from build123d import *

# Parameters (mm, degrees)
F0_W      = 43
F0_H      = 79
F0_W_2    = 28
F0_H_2    = 64
F1_DEPTH  = 22
F2_W      = 26
F2_H      = 10.2
F2_H_2    = 1.8
F2_H_3    = 5
F2_W_2    = 1
F3_DEPTH  = 100
F4_R      = 1.75
F5_DEPTH  = 100
F4_R_2    = 3
F6_DEPTH  = 2
F7_R      = 1.75
F8_DEPTH  = 2
F9_W      = 8.5
F9_H      = 20
F10_DEPTH = 20
F11_R     = 3
F12_DEPTH = 25
F13_SIZE  = 2
F14_R     = 5
F15_R     = 2


# Not quite as in the source:
# - a feature names something its author has since deleted; it is built from what else it names


with BuildPart() as f1:
    # F0 (on Top) → F1 (new body)
    with BuildSketch(Plane.XY):
        Rectangle(F0_W, F0_H)
        Rectangle(F0_W_2, F0_H_2, mode=Mode.SUBTRACT)
        Rectangle(F0_W_2, F0_H_2)
    extrude(amount=F1_DEPTH)

    # F2 (on face) → F3 (cut)
    with BuildSketch(Plane.XZ.offset(39.5)):
        with Locations((0, 16.9)):
            Rectangle(F2_W, F2_H)
        with Locations((0, 10.9)):
            Rectangle(F2_W, F2_H_2)
        with Locations((0, 7.5)):
            Rectangle(F2_W, F2_H_3)
        with Locations((-13.5, 10.9)):
            Rectangle(F2_W_2, F2_H_2)
        with Locations((13.5, 10.9)):
            Rectangle(F2_W_2, F2_H_2)
    extrude(amount=-F3_DEPTH, mode=Mode.SUBTRACT)

    # F4 (on face) → F5 (cut)
    with BuildSketch(Plane(origin=(-21.5, 0, 0), x_dir=(0, -1, 0), z_dir=(-1, 0, 0))):
        with Locations((16.5, 17)):
            Circle(F4_R)
    extrude(amount=-F5_DEPTH, mode=Mode.SUBTRACT)

    # F4 (on face) → F6 (cut)
    with BuildSketch(Plane(origin=(-21.5, 0, 0), x_dir=(0, -1, 0), z_dir=(-1, 0, 0))):
        with Locations((16.5, 17)):
            Circle(F4_R_2)
        with Locations((16.5, 17)):
            Circle(F4_R, mode=Mode.SUBTRACT)
    extrude(amount=-F6_DEPTH, mode=Mode.SUBTRACT)

    # F7 (on face) → F8 (cut)
    with BuildSketch(Plane.YZ.offset(21.5)):
        Polygon((-18.2320508076, 14), (-14.7679491924, 14), (-13.0358983849, 17), (-14.7679491924, 20), (-18.2320508076, 20), (-19.9641016151, 17), align=None)
        with Locations((-16.5, 17)):
            Circle(F7_R, mode=Mode.SUBTRACT)
    extrude(amount=-F8_DEPTH, mode=Mode.SUBTRACT)

    # F9 (on face) → F10 (join)
    with BuildSketch(Plane.XY.offset(22)):
        with Locations((17.25, -2.5)):
            Rectangle(F9_W, F9_H)
    extrude(amount=F10_DEPTH)

    # F11 (on face) → F12 (cut)
    with BuildSketch(Plane.YZ.offset(21.5)):
        with Locations((-2.5, 32)):
            Circle(F11_R)
    extrude(amount=-F12_DEPTH, mode=Mode.SUBTRACT)

    # F13
    f13_edges = [f1.edges().sort_by_distance(p)[0] for p in [
        (13, -5.5, 32),
    ]]
    chamfer(f13_edges, length=F13_SIZE)

    # F14
    f14_edges = [f1.edges().sort_by_distance(p)[0] for p in [
        (17.25, 7.5, 42),
        (17.25, -12.5, 42),
        (17.25, -12.5, 22),
        (17.25, 7.5, 22),
        (17.25, 39.5, 22),
        (17.25, -39.5, 22),
        (-17.25, -39.5, 22),
        (-17.25, 39.5, 22),
    ]]
    fillet(f14_edges, radius=F14_R)

    # F15
    f15_edges = [f1.edges().sort_by_distance(p)[0] for p in [
        (13, 0, 5),
        (-13, 0, 5),
        (21.5, 0, 0),
        (-21.5, 0, 0),
    ]]
    fillet(f15_edges, radius=F15_R)


solid = f1.part
Design review of the part built by this model. Coordinates are the model's own, in mm. A direction names the side the tool comes from. Round coordinates to 2 decimals unless told otherwise and drop trailing zeros. Write each loop counter-clockwise with the first axis right and the second up, starting at its lowest first coordinate (ties: lowest second). Pieces come first, ordered by that corner, then holes.
Item 1: Consider section B-B on z = 32. Give the boundary of the cut face in (x, y).
Item 2: Draft analysis for pull direction Z (two halves, no side actions). For faces 1 (the cylindrical face through (17.31, 6, 40.57)), 2 (the cylindrical face through (16.205, -16.272, 18.735)), 3 (the flat face through (-13, -1, 9)), state which applies: released by +Z, released by -Z, zero draft, split by the parting line, or undercut.
Item 3: Consider section C-C on x = -18. Give the boundary of the cut face in (y, z), and give its area (3 significant figures).
Item 4: For faces 4 (the flat face through (17, -26, 22)), 5 (the cylindrical face through (-20.5, -14.1, 15.2)), 6 (the cylindrical face through (-12.4, 0.55, 5.57)), 7 (the flat face through (19.5, -15, 15.7)), list the 3-axis set-ups (+Z, -Z, +X, -X, +Y, -Y) from which the entire face can be reached by the end or side of a thin tool; tool diameter is ignored.
Item 5: Wall thickness on L1, parallel to Z at x = 18, y = -2.5; L2, parallel to Y at x = 17, z = 17; L3, parallel to X at y = 26.5, z = 14.5: over which ranges is each line inside the solid? List them lowest first.
Item 6: Consider section D-D on y = 18. Give the boundary of the cut face in (x, z).
Item 7: For pin 1 Ø2.5 at (x, y) = (16, -28.5) entering from +Z; pin 2 Ø1 at (x, y) = (-4, 23) entering from +Z; pin 3 Ø3 at (y, z) = (5.5, 25) entering from -X; pin 4 Ø6.5 at (y, z) = (-16.5, 17.5) entering from -X, all flat-tipped, find the tip position at first contact; note any pin that passes through.
Item 8: Consider section A-A on y = -2.5. Give the boundary of the cut face in (x, z), and give its area (3 significant figures).
Check values:
1. outline: (13, -12.5) - (21.5, -12.5) - (21.5, -5.5) - (15, -5.5) - (13, -7.5) - close; (13, 2.5) - (15, 0.5) - (21.5, 0.5) - (21.5, 7.5) - (13, 7.5) - close
2. face 1: released by +Z
2. face 2: undercut
2. face 3: zero draft
3. outline: (-39.5, 0) - (39.5, 0) - (39.5, 17) arc R5 ccw to (34.5, 22) - (-34.5, 22) arc R5 ccw to (-39.5, 17) - close; hole circle Ø3.5 at (-16.5, 17)
3. area: 1,720 mm2
4. face 4: +Z, +X, -X, -Y
4. face 5: -X
4. face 6: +Z, +Y, -Y
4. face 7: +X
5. L1: z = 0 to 29, 35 to 42
5. L2: y = -39.5 to -18.25, -14.75 to 39.5
5. L3: x = -21.5 to -13, 13 to 21.5
6. outline: (-21.5, 2) arc R2 ccw to (-19.5, 0) - (19.5, 0) arc R2 ccw to (21.5, 2) - (21.5, 22) - (13, 22) - (13, 11.8) - (14, 11.8) - (14, 10) - (13, 10) - (13, 7) arc R2 cw to (11, 5) - (-11, 5) arc R2 cw to (-13, 7) - (-13, 10) - (-14, 10) - (-14, 11.8) - (-13, 11.8) - (-13, 22) - (-21.5, 22) - close
7. pin 1: stops at z = 22
7. pin 2: stops at z = 5
7. pin 3: stops at x = 13
7. pin 4: stops at x = -21.5
8. outline: (-21.5, 2) arc R2 ccw to (-19.5, 0) - (19.5, 0) arc R2 ccw to (21.5, 2) - (21.5, 29) - (15, 29) - (13, 27) - (13, 11.8) - (14, 11.8) - (14, 10) - (13, 10) - (13, 7) arc R2 cw to (11, 5) - (-11, 5) arc R2 cw to (-13, 7) - (-13, 10) - (-14, 10) - (-14, 11.8) - (-13, 11.8) - (-13, 22) - (-21.5, 22) - close; (13, 37) - (15, 35) - (21.5, 35) - (21.5, 42) - (13, 42) - close
8. area: 615 mm2
